from build123d import *

# Parameters (mm, degrees)
BOSS_EXTRUDE1_DEPTH     = 33
CUT_EXTRUDE1_DEPTH      = 91.853055804
CUT_EXTRUDE1_DEPTH_BACK = 10
SKETCH2_W               = 22.2275
SKETCH2_H               = 11
SKETCH3_R               = 1.5
CUT_EXTRUDE2_DEPTH      = 8


with BuildPart() as part:
    # Sketch1 → Boss-Extrude1 (new body)
    with BuildSketch(Plane.XY):
        with BuildLine():
            Line((-20.326959821, 19.197684275), (16.548040179, 19.197684275))
            Line((16.548040179, 19.197684275), (16.548040179, 14.197684275))
            Line((16.548040179, 14.197684275), (-12.326959821, 14.197684275))
            Line((-12.326959821, 14.197684275), (-12.326959821, -32.802315725))
            ThreePointArc((-12.326959821, -32.802315725), (-31.378402335, -38.048517976), (-44.551959821, -52.777315725))
            Line((-44.551959821, -52.777315725), (-44.551959821, -25.802315725))
            Line((-44.551959821, -25.802315725), (-20.326959821, -25.802315725))
            Line((-20.326959821, -25.802315725), (-20.326959821, 14.197684275))
            Line((-20.326959821, 14.197684275), (-20.326959821, 19.197684275))
        make_face()
    extrude(amount=BOSS_EXTRUDE1_DEPTH)

    # Sketch2 → Cut-Extrude1 (cut, two sides: drawn at the far end of the back side and taken through both)
    with BuildSketch(Plane(origin=(0, 19.197684275, 0), x_dir=(1, 0, 0), z_dir=(0, 1, 0)).offset(-CUT_EXTRUDE1_DEPTH_BACK)):
        with Locations((-1.213209821, -16.5)):
            Rectangle(SKETCH2_W, SKETCH2_H)
    extrude(amount=CUT_EXTRUDE1_DEPTH + CUT_EXTRUDE1_DEPTH_BACK, mode=Mode.SUBTRACT)

    # Sketch3 → Cut-Extrude2 (cut)
    with BuildSketch(Plane.ZY.offset(44.551959821)):
        with Locations((16.5, -40.777315725)):
            Circle(SKETCH3_R)
        with Locations((16.5, -30.777315725)):
            Circle(SKETCH3_R)
    extrude(amount=-CUT_EXTRUDE2_DEPTH, mode=Mode.SUBTRACT)


solid = part.part
Verification items for the finished model (mm, model axes). A direction names the side the tool comes from. Coordinates: 2 decimals unless noted, no trailing zeros. Order: outer loops, then holes, each group sorted by start corner. A loop starts at its lowest first (then second) coordinate and runs counter-clockwise, first axis right, second up.
1. Go/stop test with flat-tipped pins: pin 1 Ø5.5 at (y, z) = (16, 14) entering from -X; pin 2 Ø7.5 at (x, z) = (-36.5, 18) entering from +Y; pin 3 Ø8 at (y, z) = (-15, 21.5) entering from +X. Record where each tip stops, or that it passes through.
Results found:
pin 1: stops at x = -20.33
pin 2: stops at y = -25.8
pin 3: stops at x = -12.33
2. Set-up check for faces 5 (the face through (-1, 17, 11)), 6 (the face through (2, 14.198, 24)), 7 (the face through (-36.552, -41, 16)), 8 (the face through (-20.327, -4, 16)): record each of +Z, -Z, +X, -X, +Y, -Y from which the full face is reachable in a straight line by a thin tool's end or side.
Results found:
face 5: +Y, -Y
face 6: +Z, -Z, +X, -Y
face 7: -X
face 8: +Z, -Z, -X, +Y
3. Sectioned sample at D-D, the plane y = 1.5. Record the cut outline in (x, z).
Results found:
outline: (-20.33, 0) - (-12.33, 0) - (-12.33, 33) - (-20.33, 33) - close
4. Scan lines: line 1 (Y direction, x = -40.75, z = 16.5); line 2 (X direction, y = 15.5, z = 16); line 3 (Y direction, x = -38.5, z = 16.5). Record each from-to range of solid material in increasing order.
Results found:
line 1: y = -46.55 to -42.28, -39.28 to -32.28, -29.28 to -25.8
line 2: x = -20.33 to -12.33, 9.9 to 16.55
line 3: y = -43.89 to -42.28, -39.28 to -32.28, -29.28 to -25.8
5. Sectioned sample at B-B, the plane x = -5. Record the cut outline in (y, z), and give its area (3 significant figures).
Results found:
outline: (14.2, 0) - (19.2, 0) - (19.2, 11) - (14.2, 11) - close; (14.2, 22) - (19.2, 22) - (19.2, 33) - (14.2, 33) - close
area: 110 mm2
6. Release check for a two-part mould opening along X. For faces 1 (the face through (-40.61, -31.69, 15.31)), 2 (the face through (-36.552, -31, 16)), 3 (the face through (9.901, 17, 17)), 4 (the face through (-1, 17, 22)) record: +X half, -X half, draft (parallel to the pull), parting line (faces both ways), or undercut.
Results found:
face 1: draft
face 2: -X half
face 3: undercut
face 4: undercut
7. Sectioned sample at C-C, the plane z = 4.5. Record the cut outline in (x, y).
Results found:
outline: (-44.55, -52.78) arc R35 cw to (-12.33, -32.8) - (-12.33, 14.2) - (16.55, 14.2) - (16.55, 19.2) - (-20.33, 19.2) - (-20.33, -25.8) - (-44.55, -25.8) - close
8. Sectioned sample at A-A, the plane z = 14. Record the cut outline in (x, y), and give its area (3 significant figures).
Results found:
outline: (-44.55, -52.78) arc R35 cw to (-12.33, -32.8) - (-12.33, 19.2) - (-20.33, 19.2) - (-20.33, -25.8) - (-44.55, -25.8) - close; (9.9, 14.2) - (16.55, 14.2) - (16.55, 19.2) - (9.9, 19.2) - close
area: 797 mm2
